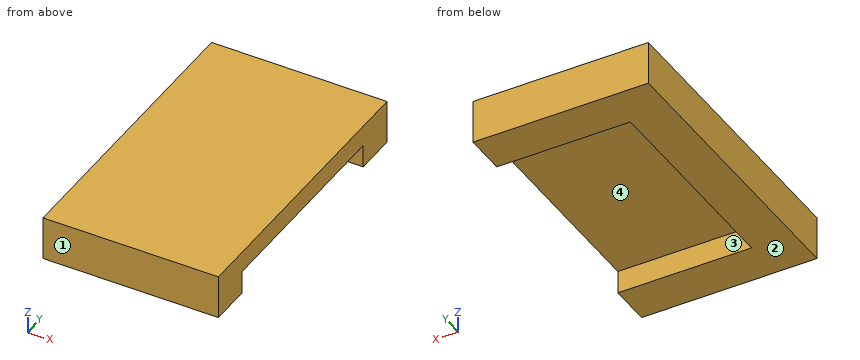
from build123d import *

# Parameters (mm, degrees)
SALIENTE_EXTRUIR1_DEPTH = 5.5
CROQUIS2_W              = 42
CROQUIS2_H              = 70.95
SALIENTE_EXTRUIR2_DEPTH = 5


with BuildPart() as part:
    # Croquis1 → Saliente-Extruir1 (new body)
    with BuildSketch(Plane.XY):
        Polygon((-16, -25.435), (-16, 25.515), (16, 25.515), (16, 35.515), (-26, 35.515), (-26, -35.435), (16, -35.435), (16, -25.435), align=None)
    extrude(amount=SALIENTE_EXTRUIR1_DEPTH)

    # Croquis2 → Saliente-Extruir2 (add)
    with BuildSketch(Plane.XY.offset(5.5)):
        with Locations((-5, 0.04)):
            Rectangle(CROQUIS2_W, CROQUIS2_H)
    extrude(amount=SALIENTE_EXTRUIR2_DEPTH)


solid = part.part
Check sheet for the modelled part. Datum: model origin and axes. Units: mm. Face numbers are marked on the shaded views. Round coordinates to 2 decimals unless told otherwise and drop trailing zeros. Order: outer loops, then holes, each group sorted by start corner. A loop starts at its lowest first (then second) coordinate and runs counter-clockwise, first axis right, second up.
Q1. Cross-section at B-B, the plane y = -13. Enter the section's corners in (x, z), plus the area to 3 significant figures.
Filled sheet:
outline: (-26, 0) - (-16, 0) - (-16, 5.5) - (16, 5.5) - (16, 10.5) - (-26, 10.5) - close
area: 265 mm2
Q2. Cross-section at C-C, the plane x = -13. Enter the section's corners in (y, z) (3 decimals).
Filled sheet:
outline: (-35.435, 0) - (-25.435, 0) - (-25.435, 5.5) - (25.515, 5.5) - (25.515, 0) - (35.515, 0) - (35.515, 10.5) - (-35.435, 10.5) - close
Q3. Depth check by flat-ended pin: P1, Ø5, axis at y = -11, z = 4.5, coming from the +X side; P2, Ø8, axis at x = -10, y = -4.5, coming from the -Z side. Enter the tip coordinate at first touch or a pass-through.
Filled sheet:
P1: stops at x = 16
P2: stops at z = 5.5
Q4. Cross-section at A-A, the plane z = 2. Enter the section's corners in (x, y) (3 decimals), plus the area to 3 significant figures.
Filled sheet:
outline: (-26, -35.435) - (16, -35.435) - (16, -25.435) - (-16, -25.435) - (-16, 25.515) - (16, 25.515) - (16, 35.515) - (-26, 35.515) - close
area: 1,350 mm2
Q5. Scan lines: L1, parallel to Y at x = 7, z = 4.75 (3 decimals); L2, parallel to Z at x = 11.5, y = 13.5; L3, parallel to X at y = -23.5, z = 2. Record each from-to range of solid material in increasing order.
Filled sheet:
L1: y = -35.435 to -25.435, 25.515 to 35.515
L2: z = 5.5 to 10.5
L3: x = -26 to -16
Q6. Draft check along Y on the marked faces 1, 2, 3 and 4. Enter one of: pulls with the +Y half, pulls with the -Y half, needs draft (parallel to the pull), parting line crosses it, or undercut.
Filled sheet:
face 1: pulls with the -Y half
face 2: needs draft
face 3: undercut
face 4: undercut
